Geometry check sheet. Reference: the model listing, model coordinates, mm. Round coordinates to 2 decimals unless told otherwise and drop trailing zeros. Write each loop counter-clockwise with the first axis right and the second up, starting at its lowest first coordinate (ties: lowest second). Pieces come first, ordered by that corner, then holes. Notation, with made-up numbers: (78, 15) - (122, 15) arc R5 ccw to (122, 21) - close; hole circle Ø3 at (53.25, -27.75). An arc over 180 degrees is marked (long way). Return JSON: item names as keys, results as strings.
```python
from build123d import *

# Parameters (mm, degrees)
SKETCH1_W           = 73.64
SKETCH1_H           = 53.01
BOARD_OUTLINE_DEPTH = 1.6
SKETCH2_R           = 1.25
NPTH_DEPTH          = 138.043199393
SKETCH3_R           = 0.405
SKETCH3_R_2         = 0.455
SKETCH3_R_3         = 0.5
SKETCH3_R_4         = 0.66
PTH_DEPTH           = 138.043199393


with BuildPart() as part:
    # Sketch1 → Board_Outline (new body)
    with BuildSketch(Plane.XY):
        with Locations((81.27, 43.015)):
            Rectangle(SKETCH1_W, SKETCH1_H)
    extrude(amount=BOARD_OUTLINE_DEPTH)

    # Sketch2 → NPTH (cut, through all)
    with BuildSketch(Plane.XY):
        with Locations((60.29, 4.82)):
            Circle(SKETCH2_R)
        with Locations((135.29, 4.82)):
            Circle(SKETCH2_R)
        with Locations((60.29, 35.82)):
            Circle(SKETCH2_R)
        with Locations((135.29, 35.82)):
            Circle(SKETCH2_R)
    extrude(amount=NPTH_DEPTH, mode=Mode.SUBTRACT)

    # Sketch3 → PTH (cut, through all)
    with BuildSketch(Plane.XY):
        with Locations((88.9, 49.53)):
            Circle(SKETCH3_R)
        with Locations((91.44, 49.53)):
            Circle(SKETCH3_R)
        with Locations((91.44, 41.91)):
            Circle(SKETCH3_R)
        with Locations((91.44, 44.45)):
            Circle(SKETCH3_R)
        with Locations((87.63, 41.91)):
            Circle(SKETCH3_R)
        with Locations((87.63, 44.45)):
            Circle(SKETCH3_R)
        with Locations((52.07, 50.8)):
            Circle(SKETCH3_R_2)
        with Locations((54.61, 50.8)):
            Circle(SKETCH3_R_2)
        with Locations((57.15, 50.8)):
            Circle(SKETCH3_R_2)
        with Locations((65.79, 35.82)):
            Circle(SKETCH3_R_3)
        with Locations((68.33, 35.82)):
            Circle(SKETCH3_R_3)
        with Locations((70.87, 35.82)):
            Circle(SKETCH3_R_3)
        with Locations((73.41, 35.82)):
            Circle(SKETCH3_R_3)
        with Locations((75.95, 35.82)):
            Circle(SKETCH3_R_3)
        with Locations((78.49, 35.82)):
            Circle(SKETCH3_R_3)
        with Locations((81.03, 35.82)):
            Circle(SKETCH3_R_3)
        with Locations((83.57, 35.82)):
            Circle(SKETCH3_R_3)
        with Locations((86.11, 35.82)):
            Circle(SKETCH3_R_3)
        with Locations((88.65, 35.82)):
            Circle(SKETCH3_R_3)
        with Locations((91.19, 35.82)):
            Circle(SKETCH3_R_3)
        with Locations((93.73, 35.82)):
            Circle(SKETCH3_R_3)
        with Locations((96.27, 35.82)):
            Circle(SKETCH3_R_3)
        with Locations((98.81, 35.82)):
            Circle(SKETCH3_R_3)
        with Locations((101.35, 35.82)):
            Circle(SKETCH3_R_3)
        with Locations((103.89, 35.82)):
            Circle(SKETCH3_R_3)
        with Locations((68.58, 53.34)):
            Circle(SKETCH3_R)
        with Locations((71.12, 53.34)):
            Circle(SKETCH3_R)
        with Locations((73.66, 53.34)):
            Circle(SKETCH3_R)
        with Locations((76.2, 53.34)):
            Circle(SKETCH3_R)
        with Locations((78.74, 53.34)):
            Circle(SKETCH3_R)
        with Locations((81.28, 53.34)):
            Circle(SKETCH3_R)
        with Locations((83.82, 53.34)):
            Circle(SKETCH3_R)
        with Locations((86.36, 53.34)):
            Circle(SKETCH3_R)
        with Locations((88.9, 53.34)):
            Circle(SKETCH3_R)
        with Locations((91.44, 53.34)):
            Circle(SKETCH3_R)
        with Locations((93.98, 53.34)):
            Circle(SKETCH3_R)
        with Locations((96.52, 53.34)):
            Circle(SKETCH3_R)
        with Locations((99.06, 53.34)):
            Circle(SKETCH3_R)
        with Locations((101.6, 53.34)):
            Circle(SKETCH3_R)
        with Locations((101.6, 60.96)):
            Circle(SKETCH3_R)
        with Locations((99.06, 60.96)):
            Circle(SKETCH3_R)
        with Locations((96.52, 60.96)):
            Circle(SKETCH3_R)
        with Locations((93.98, 60.96)):
            Circle(SKETCH3_R)
        with Locations((91.44, 60.96)):
            Circle(SKETCH3_R)
        with Locations((88.9, 60.96)):
            Circle(SKETCH3_R)
        with Locations((86.36, 60.96)):
            Circle(SKETCH3_R)
        with Locations((83.82, 60.96)):
            Circle(SKETCH3_R)
        with Locations((81.28, 60.96)):
            Circle(SKETCH3_R)
        with Locations((78.74, 60.96)):
            Circle(SKETCH3_R)
        with Locations((76.2, 60.96)):
            Circle(SKETCH3_R)
        with Locations((73.66, 60.96)):
            Circle(SKETCH3_R)
        with Locations((71.12, 60.96)):
            Circle(SKETCH3_R)
        with Locations((68.58, 60.96)):
            Circle(SKETCH3_R)
        with Locations((54.61, 63.5)):
            Circle(SKETCH3_R)
        with Locations((62.23, 63.5)):
            Circle(SKETCH3_R)
        with Locations((62.23, 59.69)):
            Circle(SKETCH3_R)
        with Locations((54.61, 59.69)):
            Circle(SKETCH3_R)
        with Locations((67.31, 49.53)):
            Circle(SKETCH3_R)
        with Locations((64.77, 49.53)):
            Circle(SKETCH3_R)
        with Locations((49.53, 64.74)):
            Circle(SKETCH3_R_4)
        with Locations((49.53, 59.72)):
            Circle(SKETCH3_R_4)
        with Locations((87.6, 24.13)):
            Circle(SKETCH3_R_4)
        with Locations((82.58, 24.13)):
            Circle(SKETCH3_R_4)
    extrude(amount=PTH_DEPTH, mode=Mode.SUBTRACT)


solid = part.part
```
(1) Section check A-A, the plane x = 60.29. Enter the section's corners in (y, z).
Response values:
{"outline": "(16.51, 0) - (34.57, 0) - (34.57, 1.6) - (16.51, 1.6) - close; (37.07, 0) - (69.52, 0) - (69.52, 1.6) - (37.07, 1.6) - close"}
(2) Material ranges on line 1 along Y through (x, z) = (93.73, 0.9); line 2 along Y through (x, z) = (88.9, 0.3) (3 decimals); line 3 along Y through (x, z) = (99.06, 1.2) (3 decimals), recorded low to high. Write a range as [from, to].
Response values:
{"line 1": "y = [16.51, 35.32], [36.32, 53.02], [53.66, 60.64], [61.28, 69.52]", "line 2": "y = [16.51, 35.387], [36.253, 49.125], [49.935, 52.935], [53.745, 60.555], [61.365, 69.52]", "line 3": "y = [16.51, 35.387], [36.253, 52.935], [53.745, 60.555], [61.365, 69.52]"}
(3) Release check for a two-part mould opening along Y. For faces 1 (the face through (81, 43, 0)), 2 (the face through (60.962, 36.874, 0.789)), 3 (the face through (81, 16.51, 1)) record: pulls with the +Y half, pulls with the -Y half, needs draft (parallel to the pull), parting line crosses it, or undercut.
Response values:
{"face 1": "needs draft", "face 2": "undercut", "face 3": "pulls with the -Y half"}
